Geometry check sheet. Reference: the model listing, model coordinates, mm. A direction names the side the tool comes from. Give positions to 0.01 mm unless a question says otherwise; leave off trailing zeros.
1. Tool access check on faces 3 (the cylindrical face through (37.257, 0.783, -8.131)), 4 (the flat face through (77, 0, -39)). Record the directions out of +Z, -Z, +X, -X, +Y, -Y that give a thin tool (end or side, any length) a straight path to the whole face; none if there is none.
2. Release check for a two-part mould opening along Z. For faces 1 (the cylindrical face through (3.515, 0.805, -2.097)), 2 (the flat face through (77, 1.588, -18)) record: +Z half, -Z half, draft (parallel to the pull), parting line (faces both ways), or undercut.
3. Go/stop test with flat-tipped pins: pin 1 Ø0.6 at (x, z) = (53, -6) entering from +Y; pin 2 Ø1.4 at (x, z) = (3.175, -3.175) entering from -Y. Record where each tip stops, or that it passes through.
4. Material ranges on L1, parallel to Z at x = 14, y = 1.4; L2, parallel to X at y = 0.1, z = -31.5; L3, parallel to X at y = 1.25, z = -21.5, recorded low to high.
5. Cross-section at C-C, the plane y = 1.1. State how many separate pieces and enclosed holes the cut face has, plus the area to 3 significant figures.
from build123d import *

# Parameters (mm, degrees)
SKETCH1_W           = 127
SKETCH1_H           = 63.5
BOSS_EXTRUDE1_DEPTH = 1.5875
SKETCH2_R           = 1.1303
CUT_EXTRUDE1_DEPTH  = 142.999190689
CUT_EXTRUDE2_DEPTH  = 1.5875
CUT_EXTRUDE3_START  = -1.5875
CUT_EXTRUDE3_DEPTH  = 1.5875
SKETCH3_R           = 1.016
CUT_EXTRUDE4_DEPTH  = 0.0254


# Read off the part's stored shape, not the designer's step: Cut-Extrude3
with BuildPart() as part:
    # Sketch1 → Boss-Extrude1 (new body)
    with BuildSketch(Plane(origin=(0, 0, 0), x_dir=(1, 0, 0), z_dir=(0, 1, 0))):
        with Locations((63.5, 31.75)):
            Rectangle(SKETCH1_W, SKETCH1_H)
    extrude(amount=BOSS_EXTRUDE1_DEPTH)

    # Sketch2 → Cut-Extrude1 (cut, through all)
    with BuildSketch(Plane(origin=(0, 1.5875, 0), x_dir=(1, 0, 0), z_dir=(0, 1, 0))):
        with Locations(Location((3.175, 60.325, 0), (0, 0, 270))):
            Circle(SKETCH2_R)
        with Locations(Location((3.175, 3.175, 0), (0, 0, 270))):
            Circle(SKETCH2_R)
        with Locations(Location((123.825, 3.175, 0), (0, 0, 90))):
            Circle(SKETCH2_R)
        with Locations(Location((123.825, 60.325, 0), (0, 0, 90))):
            Circle(SKETCH2_R)
    extrude(amount=-CUT_EXTRUDE1_DEPTH, mode=Mode.SUBTRACT)

    # Sketch4 → Cut-Extrude2 (cut)
    with BuildSketch(Plane(origin=(0, 1.5875, 0), x_dir=(1, 0, 0), z_dir=(0, 1, 0))):
        with BuildLine():
            Line((72.832403955, 28.767596045), (98.232403955, 54.167596045))
            ThreePointArc((98.232403955, 54.167596045), (104.967596045, 54.167596045), (104.967596045, 47.432403955))
            Line((104.967596045, 47.432403955), (79.567596045, 22.032403955))
            ThreePointArc((79.567596045, 22.032403955), (72.832403955, 22.032403955), (72.832403955, 28.767596045))
        make_face()
        with BuildLine():
            Line((101.6, 55.5625), (127, 55.5625))
            ThreePointArc((127, 55.5625), (131.7625, 50.8), (127, 46.0375))
            Line((127, 46.0375), (101.6, 46.0375))
            ThreePointArc((101.6, 46.0375), (96.8375, 50.8), (101.6, 55.5625))
        make_face()
    extrude(amount=-CUT_EXTRUDE2_DEPTH, mode=Mode.SUBTRACT)

    # Cut-Extrude3 outline → Cut-Extrude3 (cut)
    with BuildSketch(Plane(origin=(0, 1.5875, 0), x_dir=(-1, 0, 0), z_dir=(0, 1, 0)).offset(CUT_EXTRUDE3_START)):
        with BuildLine():
            ThreePointArc((-61.274445986, -48.41875), (-61.274445986, -53.18125), (-57.15, -55.5625))
            Line((-57.15, -55.5625), (-12.489472227, -55.5625))
            ThreePointArc((-12.489472227, -55.5625), (-10.065969168, -54.899760868), (-8.316964929, -53.095994141))
            Line((-8.316964929, -53.095994141), (-5.499068963, -48.1499644))
            ThreePointArc((-5.499068963, -48.1499644), (-4.790682084, -46.79307626), (-4.549320114, -45.281553255))
            Line((-4.549320114, -45.281553255), (-4.650233894, -12.25819272))
            ThreePointArc((-4.650233894, -12.25819272), (-6.050264926, -8.900008545), (-9.412711658, -7.510246043))
            Line((-9.412711658, -7.510246043), (-34.906279557, -7.510246043))
            ThreePointArc((-34.906279557, -7.510246043), (-37.287529557, -8.148300057), (-39.030725542, -9.891496043))
            Line((-39.030725542, -9.891496043), (-61.274445986, -48.41875))
        make_face()
    extrude(amount=CUT_EXTRUDE3_DEPTH, mode=Mode.SUBTRACT)

    # Sketch3 → Cut-Extrude4 (cut)
    with BuildSketch(Plane(origin=(0, 1.5875, 0), x_dir=(1, 0, 0), z_dir=(0, 1, 0))):
        with Locations(Location((63.5, 6.35, 0), (0, 0, 270))):
            Circle(SKETCH3_R)
        with Locations(Location((66.04, 6.35, 0), (0, 0, 270))):
            Circle(SKETCH3_R)
        with Locations(Location((68.58, 6.35, 0), (0, 0, 270))):
            Circle(SKETCH3_R)
        with Locations(Location((71.12, 6.35, 0), (0, 0, 270))):
            Circle(SKETCH3_R)
        with Locations(Location((73.66, 6.35, 0), (0, 0, 270))):
            Circle(SKETCH3_R)
        with Locations(Location((60.96, 6.35, 0), (0, 0, 270))):
            Circle(SKETCH3_R)
        with Locations(Location((58.42, 6.35, 0), (0, 0, 270))):
            Circle(SKETCH3_R)
        with Locations(Location((55.88, 6.35, 0), (0, 0, 270))):
            Circle(SKETCH3_R)
        with Locations(Location((53.34, 6.35, 0), (0, 0, 270))):
            Circle(SKETCH3_R)
        with BuildLine():
            Line((5.715, 50.8), (5.715, 12.7))
            ThreePointArc((5.715, 12.7), (3.81, 10.795), (1.905, 12.7))
            Line((1.905, 12.7), (1.905, 50.8))
            ThreePointArc((1.905, 50.8), (3.81, 52.705), (5.715, 50.8))
        make_face()
        with BuildLine():
            Line((50.8, 57.634853503), (12.7, 57.634853503))
            ThreePointArc((12.7, 57.634853503), (10.795, 59.539853503), (12.7, 61.444853503))
            Line((12.7, 61.444853503), (50.8, 61.444853503))
            ThreePointArc((50.8, 61.444853503), (52.705, 59.539853503), (50.8, 57.634853503))
        make_face()
        with BuildLine():
            Line((76.2, 57.634853503), (114.3, 57.634853503))
            ThreePointArc((114.3, 57.634853503), (116.205, 59.539853503), (114.3, 61.444853503))
            Line((114.3, 61.444853503), (76.2, 61.444853503))
            ThreePointArc((76.2, 61.444853503), (74.295, 59.539853503), (76.2, 57.634853503))
        make_face()
        with BuildLine():
            Line((125.095, 44.45), (125.095, 12.7))
            ThreePointArc((125.095, 12.7), (123.19, 10.795), (121.285, 12.7))
            Line((121.285, 12.7), (121.285, 44.45))
            ThreePointArc((121.285, 44.45), (123.19, 46.355), (125.095, 44.45))
        make_face()
    extrude(amount=-CUT_EXTRUDE4_DEPTH, mode=Mode.SUBTRACT)


solid = part.part
Result:
1. face 3: +Y, -Y
1. face 4: +Z, -Z, +X, -X, -Y
2. face 1: undercut
2. face 2: draft
3. pin 1: stops at y = 1.56
3. pin 2: passes through
4. L1: z = -63.5 to -55.56, -7.51 to 0
4. L2: x = 0 to 4.59, 51.51 to 75.56, 89.04 to 127
4. L3: x = 0 to 4.62, 45.73 to 73.47, 78.93 to 127
5. separate pieces: 1
5. enclosed holes: 5
5. area: 5,220 mm2
